```python
from build123d import *

# Parameters (mm, degrees)
SKETCH1_R           = 2.275
SKETCH1_R_2         = 4
SKETCH1_W           = 14
SKETCH1_H           = 14
BOSS_EXTRUDE1_DEPTH = 3
SKETCH2_R           = 1.5
SKETCH2_R_2         = 4
SKETCH2_W           = 37.05
SKETCH2_H           = 56.1
SKETCH2_W_2         = 18
SKETCH2_H_2         = 18
BOSS_EXTRUDE2_DEPTH = 2
SKETCH3_W           = 14.2
SKETCH3_H           = 17.5
CUT_EXTRUDE1_DEPTH  = 4.5
SKETCH4_W           = 61.5
SKETCH4_H           = 11.425
CUT_EXTRUDE2_DEPTH  = 171.146995272
FILLET1_R           = 0.5
FILLET2_R           = 2


with BuildPart() as part:
    # Sketch1 → Boss-Extrude1 (new body)
    with BuildSketch(Plane(origin=(0, 0, 0), x_dir=(1, 0, 0), z_dir=(0, 1, 0))):
        with BuildLine():
            Line((0.5, 0), (154.5, 0))
            ThreePointArc((154.5, 0), (154.853553391, 0.146446609), (155, 0.5))
            Line((155, 0.5), (155, 69.5))
            ThreePointArc((155, 69.5), (154.853553391, 69.853553391), (154.5, 70))
            Line((154.5, 70), (0.5, 70))
            ThreePointArc((0.5, 70), (0.146446609, 69.853553391), (0, 69.5))
            Line((0, 69.5), (0, 0.5))
            ThreePointArc((0, 0.5), (0.146446609, 0.146446609), (0.5, 0))
        make_face()
        with Locations(Location((4, 66, 0), (0, 0, 270))):
            Circle(SKETCH1_R, mode=Mode.SUBTRACT)
        with Locations(Location((4, 4, 0), (0, 0, 90))):
            Circle(SKETCH1_R, mode=Mode.SUBTRACT)
        with Locations(Location((151, 4, 0), (0, 0, 270))):
            Circle(SKETCH1_R, mode=Mode.SUBTRACT)
        with Locations(Location((151, 66, 0), (0, 0, 90))):
            Circle(SKETCH1_R, mode=Mode.SUBTRACT)
        with Locations(Location((82.2625, 25.475, 0), (0, 0, 270))):
            Circle(SKETCH1_R, mode=Mode.SUBTRACT)
        with Locations(Location((120.3625, 25.475, 0), (0, 0, 270))):
            Circle(SKETCH1_R, mode=Mode.SUBTRACT)
        with Locations(Location((139.4125, 55.075, 0), (0, 0, 270))):
            Circle(SKETCH1_R_2, mode=Mode.SUBTRACT)
        with Locations((15.5875, 54.05)):
            Rectangle(SKETCH1_W, SKETCH1_H, mode=Mode.SUBTRACT)
        with Locations((34.6375, 54.05)):
            Rectangle(SKETCH1_W, SKETCH1_H, mode=Mode.SUBTRACT)
        with Locations((34.6375, 35)):
            Rectangle(SKETCH1_W, SKETCH1_H, mode=Mode.SUBTRACT)
        with Locations((34.6375, 15.95)):
            Rectangle(SKETCH1_W, SKETCH1_H, mode=Mode.SUBTRACT)
        with Locations((15.5875, 35)):
            Rectangle(SKETCH1_W, SKETCH1_H, mode=Mode.SUBTRACT)
        with Locations((15.5875, 15.95)):
            Rectangle(SKETCH1_W, SKETCH1_H, mode=Mode.SUBTRACT)
        with Locations((101.3125, 25.475)):
            Rectangle(SKETCH1_W, SKETCH1_H, mode=Mode.SUBTRACT)
        with Locations((63.2125, 25.475)):
            Rectangle(SKETCH1_W, SKETCH1_H, mode=Mode.SUBTRACT)
        with Locations((139.4125, 25.475)):
            Rectangle(SKETCH1_W, SKETCH1_H, mode=Mode.SUBTRACT)
    extrude(amount=-BOSS_EXTRUDE1_DEPTH)

    # Sketch2 → Boss-Extrude2 (add)
    with BuildSketch(Plane(origin=(0, -3, 0), x_dir=(-1, 0, 0), z_dir=(0, -1, 0))):
        with BuildLine():
            Line((-0.5, 70), (-154.5, 70))
            ThreePointArc((-154.5, 70), (-154.853553391, 69.853553391), (-155, 69.5))
            Line((-155, 69.5), (-155, 0.5))
            ThreePointArc((-155, 0.5), (-154.853553391, 0.146446609), (-154.5, 0))
            Line((-154.5, 0), (-0.5, 0))
            ThreePointArc((-0.5, 0), (-0.146446609, 0.146446609), (0, 0.5))
            Line((0, 0.5), (0, 69.5))
            ThreePointArc((0, 69.5), (-0.146446609, 69.853553391), (-0.5, 70))
        make_face()
        with Locations(Location((-4, 66, 0), (0, 0, 270))):
            Circle(SKETCH2_R, mode=Mode.SUBTRACT)
        with Locations(Location((-4, 4, 0), (0, 0, 270))):
            Circle(SKETCH2_R, mode=Mode.SUBTRACT)
        with Locations(Location((-151, 4, 0), (0, 0, 270))):
            Circle(SKETCH2_R, mode=Mode.SUBTRACT)
        with Locations(Location((-151, 66, 0), (0, 0, 270))):
            Circle(SKETCH2_R, mode=Mode.SUBTRACT)
        with Locations(Location((-82.2625, 25.475, 0), (0, 0, 270))):
            Circle(SKETCH2_R, mode=Mode.SUBTRACT)
        with Locations(Location((-120.3625, 25.475, 0), (0, 0, 270))):
            Circle(SKETCH2_R, mode=Mode.SUBTRACT)
        with Locations(Location((-139.4125, 55.075, 0), (0, 0, 270))):
            Circle(SKETCH2_R_2, mode=Mode.SUBTRACT)
        with Locations((-25.1125, 35)):
            Rectangle(SKETCH2_W, SKETCH2_H, mode=Mode.SUBTRACT)
        with Locations((-63.2125, 25.475)):
            Rectangle(SKETCH2_W_2, SKETCH2_H_2, mode=Mode.SUBTRACT)
        with Locations((-101.3125, 25.475)):
            Rectangle(SKETCH2_W_2, SKETCH2_H_2, mode=Mode.SUBTRACT)
        with Locations((-139.4125, 25.475)):
            Rectangle(SKETCH2_W_2, SKETCH2_H_2, mode=Mode.SUBTRACT)
    extrude(amount=BOSS_EXTRUDE2_DEPTH)

    # Sketch3 → Cut-Extrude1 (cut)
    with BuildSketch(Plane(origin=(0, -5, 0), x_dir=(-1, 0, 0), z_dir=(0, -1, 0))):
        with Locations((-139.4125, 55.075)):
            Rectangle(SKETCH3_W, SKETCH3_H)
    extrude(amount=-CUT_EXTRUDE1_DEPTH, mode=Mode.SUBTRACT)

    # Sketch4 → Cut-Extrude2 (cut, through all)
    with BuildSketch(Plane(origin=(0, 0, 0), x_dir=(1, 0, 0), z_dir=(0, 1, 0))):
        with Locations((101.3125, 5.7125)):
            Rectangle(SKETCH4_W, SKETCH4_H)
    extrude(amount=-CUT_EXTRUDE2_DEPTH, mode=Mode.SUBTRACT)

    # Fillet1
    fillet1_edges = [part.edges().sort_by_distance(p)[0] for p in [
        (0, 0, -35),
        (0.146446609, 0, -69.853553391),
        (77.5, 0, -70),
        (154.853553391, 0, -69.853553391),
        (143.28125, 0, 0),
        (132.0625, -2.5, 0),
        (70.5625, -2.5, 0),
        (155, 0, -35),
        (154.853553391, 0, -0.146446609),
        (35.53125, 0, 0),
        (0.146446609, 0, -0.146446609),
    ]]
    fillet(fillet1_edges, radius=FILLET1_R)

    # Fillet2
    fillet2_edges = [part.edges().sort_by_distance(p)[0] for p in [
        (70.5625, -2.5, -11.425),
        (132.0625, -2.5, -11.425),
    ]]
    fillet(fillet2_edges, radius=FILLET2_R)


solid = part.part
```
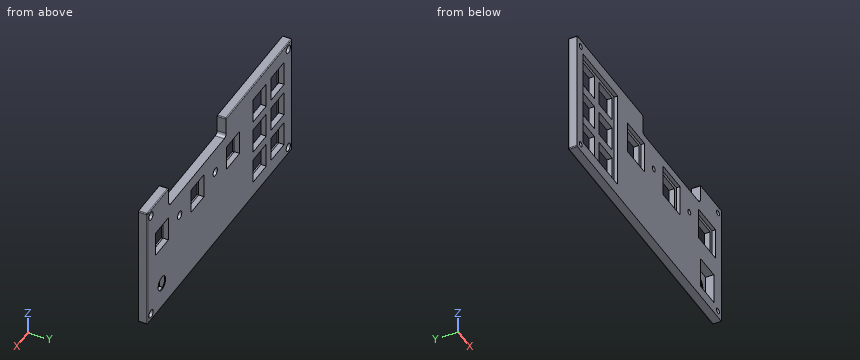
Source: CAD feature listing. Evaluate the final solid. Frame: model axes, mm. Give positions to 0.01 mm unless a question says otherwise; leave off trailing zeros. Loops run counter-clockwise (first coordinate to the right, second up) from the corner with the lowest first, then second, coordinate; pieces in that order, holes last. Notation, with made-up numbers: (86, 27.5) -> (115, 27.5) arc R17 cw to (115, 50.5) -> close; hole circle Ø2 at (12.25, -21). An arc over 180 degrees is marked (long way). Put each result on its own line as item: value. Start each with the question number.
1) Contact query for flat-ended pins moving along their axis: P1, Ø18.5, axis at x = 34, z = -35, coming from the -Y side; P2, Ø3.5, axis at x = 120.36, z = -25.48, coming from the +Y side. Output: stop coordinate, or through.
2) Cut plane C-C (x = 59.5). Return loops of the section in (y, z) (3 decimals).
3) Material intervals for probe 1 along Z at (x, y) = (151, -1.4) (3 decimals); probe 2 along X at (y, z) = (-3.1, -54); probe 3 along X at (y, z) = (-0.8, -17.5), sorted ascending.
4) Cut plane D-D (z = -4). Return loops of the section in (x, y) (1 decimal).
5) Cut plane B-B (z = -66). Return loops of the section in (x, y) (3 decimals).
6) Cut plane A-A (x = 4). Return loops of the section in (y, z) (3 decimals), then the cut area to 3 significant figures.
Results are:
1. P1: stops at y = -3
1. P2: stops at y = -3
2. outline: (-5, -70) -> (-0.5, -70) arc R0.5 ccw to (0, -69.5) -> (0, -32.475) -> (-3, -32.475) -> (-3, -34.475) -> (-5, -34.475) -> close; (-5, -16.475) -> (-3, -16.475) -> (-3, -18.475) -> (0, -18.475) -> (0, -0.5) arc R0.5 ccw to (-0.5, 0) -> (-5, 0) -> close
3. probe 1: z = -70 to -68.275, -63.725 to -6.275, -1.725 to 0
3. probe 2: x = 0 to 6.59, 43.64 to 132.31, 146.51 to 155
3. probe 3: x = 0 to 8.59, 22.59 to 27.64, 41.64 to 155
4. outline: (0, -5) -> (2.5, -5) -> (2.5, -3) -> (1.7, -3) -> (1.7, 0) -> (0.5, 0) arc R0.5 ccw to (0, -0.5) -> close; (5.5, -5) -> (70.6, -5) -> (70.6, 0) -> (6.3, 0) -> (6.3, -3) -> (5.5, -3) -> close; (132.1, -5) -> (149.5, -5) -> (149.5, -3) -> (148.7, -3) -> (148.7, 0) -> (132.1, 0) -> close; (152.5, -5) -> (155, -5) -> (155, -0.5) arc R0.5 ccw to (154.5, 0) -> (153.3, 0) -> (153.3, -3) -> (152.5, -3) -> close
5. outline: (0, -5) -> (2.5, -5) -> (2.5, -3) -> (1.725, -3) -> (1.725, 0) -> (0.5, 0) arc R0.5 ccw to (0, -0.5) -> close; (5.5, -5) -> (149.5, -5) -> (149.5, -3) -> (148.725, -3) -> (148.725, 0) -> (6.275, 0) -> (6.275, -3) -> (5.5, -3) -> close; (152.5, -5) -> (155, -5) -> (155, -0.5) arc R0.5 ccw to (154.5, 0) -> (153.275, 0) -> (153.275, -3) -> (152.5, -3) -> close
6. outline: (-5, -70) -> (-0.5, -70) arc R0.5 ccw to (0, -69.5) -> (0, -68.275) -> (-3, -68.275) -> (-3, -67.5) -> (-5, -67.5) -> close; (-5, -64.5) -> (-3, -64.5) -> (-3, -63.725) -> (0, -63.725) -> (0, -6.275) -> (-3, -6.275) -> (-3, -5.5) -> (-5, -5.5) -> close; (-5, -2.5) -> (-3, -2.5) -> (-3, -1.725) -> (0, -1.725) -> (0, -0.5) arc R0.5 ccw to (-0.5, 0) -> (-5, 0) -> close
6. area: 311 mm2
